The model under review builds one solid part; all positions refer to its coordinate system, in mm. A direction names the side the tool comes from. Give positions to 0.01 mm unless a question says otherwise; leave off trailing zeros. Write each loop counter-clockwise with the first axis right and the second up, starting at its lowest first coordinate (ties: lowest second). Pieces come first, ordered by that corner, then holes. Notation, with made-up numbers: (68, -15.5) -> (102, -15.5) arc R21 ccw to (102, 15.5) -> close; hole circle Ø2 at (12, -12). An arc over 180 degrees is marked (long way). Use CSV: the item, a comma, the result in double quotes.
```python
from build123d import *

# Parameters (mm, degrees)
SKETCH_1_R          = 2
EXTRUDE_1_DEPTH     = 0.4
SKETCH_2_R          = 1
EXTRUDE_2_DEPTH     = 18
CHAMFER_1_SIZE      = 0.2
CUT_EXTRUDE_1_DEPTH = 0.8
FILLET_2_R          = 0.3


with BuildPart() as part:
    # 草图1 → 凸台-拉伸1 (new body, symmetric)
    with BuildSketch(Plane.XY):
        Circle(SKETCH_1_R)
    extrude(amount=EXTRUDE_1_DEPTH, both=True)

    # 草图2 → 凸台-拉伸2 (add)
    with BuildSketch(Plane(origin=(0, 0, -0.4), x_dir=(-1, 0, 0), z_dir=(0, 0, -1))):
        Circle(SKETCH_2_R)
    extrude(amount=EXTRUDE_2_DEPTH)

    # 倒角1
    chamfer_1_edges = [part.edges().sort_by_distance(p)[0] for p in [
        (1, 0, -18.4),
    ]]
    chamfer(chamfer_1_edges, length=CHAMFER_1_SIZE)

    # 草图3 → 切除-拉伸1 (cut)
    with BuildSketch(Plane.XY.offset(0.4)):
        Polygon((0.75055535, 0), (0.375277675, 0.65), (-0.375277675, 0.65), (-0.75055535, 0), (-0.375277675, -0.65), (0.375277675, -0.65), align=None)
    extrude(amount=-CUT_EXTRUDE_1_DEPTH, mode=Mode.SUBTRACT)

    # 圆角2
    fillet_2_edges = [part.edges().sort_by_distance(p)[0] for p in [
        (-2, 0, -0.4),
        (-2, 0, 0.4),
    ]]
    fillet(fillet_2_edges, radius=FILLET_2_R)


solid = part.part
```
Q1. Machinability: for faces 4 (the flat face through (0, 0, -18.4)), 5 (the flat face through (1, -1, -0.4)), which of the approach directions +Z, -Z, +X, -X, +Y, -Y give a long, thin tool a straight path to every point of the face, cutting with its end or side? Answer none if there is none.
Derived:
face 4,"-Z, +X, -X, +Y, -Y"
face 5,"-Z"
Q2. Insertion check: pin 1 (2 mm diameter, centred on x = 1.5, z = -2.5, fed in from +Y); pin 2 (1 mm diameter, centred on y = -1, z = -3, fed in from +X); pin 3 (1.5 mm diameter, centred on x = 0, y = 0.5, fed in from +Z). Each pin has a flat end and moves straight along its axis. Give the tip position at first contact, or say it passes through.
Derived:
pin 1,"stops at y = 0.87"
pin 2,"stops at x = 0.87"
pin 3,"stops at z = 0.4"
Q3. The part is to be moulded in two halves that separate along X. For faces 1 (the flat face through (0, -1, 0.4)), 2 (the cylindrical face through (0, -1, -9)), 3 (the flat face through (0, 0, -0.4)), say which applies: pulls with the +X half, pulls with the -X half, needs draft (parallel to the pull), parting line crosses it, or undercut.
Derived:
face 1,"needs draft"
face 2,"parting line crosses it"
face 3,"undercut"
Q4. To check wall thickness, follow probe 1 along Z at (x, y) = (-0.75, -0.8); probe 2 along Y at (x, z) = (0.6, -2); probe 3 along Z at (x, y) = (-0.55, -0.15). State the ranges of each line that lie inside material, in increasing order.
Derived:
probe 1,"z = -0.4 to 0.4"
probe 2,"y = -0.8 to 0.8"
probe 3,"z = -18.4 to -0.4"
Q5. Consider section A-A (x = 0). Write out the cut boundary in (y, z), then the cut area to 3 significant figures.
Derived:
outline,"(-2, -0.1) arc R0.3 ccw to (-1.7, -0.4) -> (-1, -0.4) -> (-1, -18.2) -> (-0.8, -18.4) -> (0.8, -18.4) -> (1, -18.2) -> (1, -0.4) -> (1.7, -0.4) arc R0.3 ccw to (2, -0.1) -> (2, 0.1) arc R0.3 ccw to (1.7, 0.4) -> (0.65, 0.4) -> (0.65, -0.4) -> (-0.65, -0.4) -> (-0.65, 0.4) -> (-1.7, 0.4) arc R0.3 ccw to (-2, 0.1) -> close"
area,"38.0 mm2"
Q6. Consider section B-B (z = -6). Write out the cut boundary in (x, y), then the cut area to 3 significant figures.
Derived:
outline,"circle Ø2 at (0, 0)"
area,"3.14 mm2"
